The model under review builds one solid part; all positions refer to its coordinate system, in mm. A direction names the side the tool comes from. Give positions to 0.01 mm unless a question says otherwise; leave off trailing zeros. Write each loop counter-clockwise with the first axis right and the second up, starting at its lowest first coordinate (ties: lowest second). Pieces come first, ordered by that corner, then holes. Notation, with made-up numbers: (81.25, -16) - (101.25, -16) arc R30 ccw to (101.25, 17) - close; hole circle Ø7 at (68.5, 16.5). An arc over 180 degrees is marked (long way). Write item = value, one per line.
```python
from build123d import *

# Parameters (mm, degrees)
SKETCH1_W           = 60
SKETCH1_H           = 60
BOSS_EXTRUDE1_DEPTH = 20
CUT_EXTRUDE1_DEPTH  = 60
CHAMFER1_SIZE       = 5
SKETCH6_R           = 3
CUT_EXTRUDE2_DEPTH  = 59.309518948
SKETCH9_R           = 12.5
CUT_EXTRUDE4_DEPTH  = 71


with BuildPart() as part:
    # Sketch1 → Boss-Extrude1 (new, symmetric)
    with BuildSketch(Plane.XY):
        Rectangle(SKETCH1_W, SKETCH1_H)
    extrude(amount=BOSS_EXTRUDE1_DEPTH, both=True)

    # Sketch5 → Cut-Extrude1 (cut)
    with BuildSketch(Plane.XZ.offset(30)):
        with BuildLine():
            ThreePointArc((30, 0), (24.142135624, -14.142135624), (10, -20))
            Line((10, -20), (30, -20))
            Line((30, -20), (30, 0))
        make_face()
        with BuildLine():
            Line((30, 20), (10.000000023, 20))
            ThreePointArc((10.000000023, 20), (24.142135632, 14.142135615), (30, 0))
            Line((30, 0), (30, 20))
        make_face()
        with BuildLine():
            ThreePointArc((-30, -1.4e-08), (-24.142135621, 14.142135627), (-9.999999977, 20))
            Line((-9.999999977, 20), (-30, 20))
            Line((-30, 20), (-30, -1.4e-08))
        make_face()
        with BuildLine():
            Line((-30, -20), (-10, -20))
            ThreePointArc((-10, -20), (-24.142135619, -14.142135629), (-30, -1.4e-08))
            Line((-30, -1.4e-08), (-30, -20))
        make_face()
    extrude(amount=-CUT_EXTRUDE1_DEPTH, mode=Mode.SUBTRACT)

    # Chamfer1
    chamfer1_edges = [part.edges().sort_by_distance(p)[0] for p in [
        (0, 30, -20),
        (30, 30, -1.2e-08),
        (-30, 30, 1.2e-08),
        (2.3e-08, 30, 20),
    ]]
    chamfer(chamfer1_edges, length=CHAMFER1_SIZE)

    # Sketch6 → Cut-Extrude2 (cut, through all)
    with BuildSketch(Plane(origin=(0, 0, -20), x_dir=(-1, 0, 0), z_dir=(0, 0, -1))):
        Circle(SKETCH6_R)
    extrude(amount=-CUT_EXTRUDE2_DEPTH, mode=Mode.SUBTRACT)

    # Sketch9 → Cut-Extrude4 (cut, through all)
    with BuildSketch(Plane.XZ.offset(30)):
        with Locations((-7.499382611, 0)):
            Circle(SKETCH9_R)
        with Locations((7.499382611, 0)):
            Circle(SKETCH9_R)
        with BuildLine():
            ThreePointArc((0, 10.000463012), (3.546901596, 11.858663239), (7.499382611, 12.5))
            Line((7.499382611, 12.5), (-7.499382623, 12.5))
            ThreePointArc((-7.499382623, 12.5), (-3.546901601, 11.858663241), (0, 10.000463012))
        make_face()
        with BuildLine():
            Line((-7.499382656, -12.5), (7.499382577, -12.5))
            ThreePointArc((7.499382577, -12.5), (3.54690158, -11.858663234), (0, -10.000463012))
            ThreePointArc((0, -10.000463012), (-3.546901617, -11.858663246), (-7.499382656, -12.5))
        make_face()
    extrude(amount=-CUT_EXTRUDE4_DEPTH, mode=Mode.SUBTRACT)


solid = part.part
```
1. Draft analysis for pull direction Z (two halves, no side actions). For faces 1 (the flat face through (0, -30, -13)), 2 (the cylindrical face through (20, 0, 0)), 3 (the flat face through (0, 27, -18)), state which applies: +Z half, -Z half, draft (parallel to the pull), parting line (faces both ways), or undercut.
Findings below:
face_1 = draft
face_2 = undercut
face_3 = -Z half
2. Insertion check: P1, Ø8, axis at y = -19.5, z = -12.5, coming from the +X side. The pin has a flat end and moves straight along its axis. Give the tip position at first contact, or say it passes through.
Findings below:
P1 = 28.1
3. Take a section at B-B on y = 17.5. Give the boundary of the cut face in (x, z).
Findings below:
outline = (-10, -20) - (10, -20) arc R20 ccw to (10, 20) - (-10, 20) arc R20 ccw to start; hole (-7.5, -12.5) - (7.5, -12.5) arc R12.5 ccw to (7.5, 12.5) - (-7.5, 12.5) arc R12.5 ccw to start
4. Machinability: for faces 4 (the flat face through (0, 27, 18)), 5 (the flat face through (3.2, -0.4, -12.5)), which of the approach directions +Z, -Z, +X, -X, +Y, -Y give a long, thin tool a straight path to every point of the face, cutting with its end or side? Answer none if there is none.
Findings below:
face_4 = +Z, +X, -X, +Y
face_5 = +Y, -Y
5. For line 1 (Z direction, x = 5.5, y = 10); line 2 (Z direction, x = -16.5, y = -16.5); line 3 (X direction, y = -14.5, z = -1.5), list the stretches that pass through material, from the lowest coordinate up. Write a range as from..to.
Findings below:
line_1 = -20..-12.5, 12.5..20
line_2 = -18.91..-8.67, 8.67..18.91
line_3 = -29.94..-19.91, 19.91..29.94
6. Take a section at C-C on y = 0. Give the boundary of the cut face in (x, z).
Findings below:
outline = (-10, -20) - (-3, -20) - (-3, -12.5) - (-7.5, -12.5) arc R12.5 cw to (-7.5, 12.5) - (-3, 12.5) - (-3, 20) - (-10, 20) arc R20 ccw to start; (3, -20) - (10, -20) arc R20 ccw to (10, 20) - (3, 20) - (3, 12.5) - (7.5, 12.5) arc R12.5 cw to (7.5, -12.5) - (3, -12.5) - close
7. Take a section at A-A on x = 4. Give the boundary of the cut face in (y, z), and give its area (3 significant figures).
Findings below:
outline = (-30, -20) - (25, -20) - (30, -15) - (30, -12.5) - (-30, -12.5) - close; (-30, 12.5) - (30, 12.5) - (30, 15) - (25, 20) - (-30, 20) - close
area = 875 mm²
